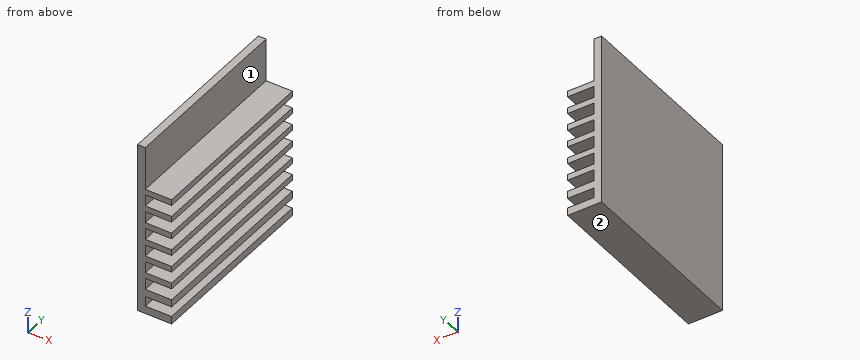
Autodesk Inventor part; units mm, degrees
ref_plane "YZ Plane" through (0, 0, 0) normal (1, 0, 0) x (0, 1, 0)
ref_plane "XZ Plane" through (0, 0, 0) normal (0, 1, 0) x (-1, 0, 0)
ref_plane "XY Plane" through (0, 0, 0) normal (0, 0, 1) x (1, 0, 0)
sketch "Sketch1" plane through (0, 0, 0) normal (0, 1, 0) x (-1, 0, 0)
  line L0 (-10, -20) -> (10, -20)
  line L1 (10, -20) -> (10, 20)
  line L2 (10, 20) -> (-10, 20)
  line L3 (-10, 20) -> (-10, -20)
  line L4 (-10, -20) -> (10, 20) construction
  line L5 (10, -20) -> (-10, 20) construction
  point P0 (0, 0)
  dimension "d0" = 20
  dimension "d1" = 40
extrude "Extrusion1" add sketch "Sketch1" along normal blind 40
sketch "Sketch2" plane through (0, 0, 0) normal (0, -1, 0) x (1, 0, 0)
  line L0 (10, -20) -> (-10, -20)
  line L1 (10, 20) -> (10, -20)
  line L2 (-10, 20) -> (10, 20)
  line L3 (-10, -20) -> (-10, 20)
  line L4 (10, 20) -> (10, -20)
  line L5 (10, 18.3) -> (-5.8, 18.3)
  line L6 (-5.8, 18.3) -> (-5.8, 16.1)
  line L7 (-5.8, 16.1) -> (10, 16.1)
  line L8 (10, 16.1) -> (10, 18.3)
  point P0 (0, 0)
  dimension "d4" = 1.7
  dimension "d5" = 4.2
  dimension "d6" = 2.2
extrude "Extrusion2" cut sketch "Sketch2" against normal through all contours L7 L6 L5 L1
mirror "Mirror1" about plane through (0, 0, 0) normal (0, 0, 1) of "Extrusion2"
sketch "Sketch3" plane through (0, 0, 0) normal (0, -1, 0) x (1, 0, 0)
  line L0 (-5.8, -16.1) -> (10, -16.1)
  line L1 (10, 16.1) -> (10, -16.1)
  line L2 (10, 16.1) -> (-5.8, 16.1)
  line L3 (-5.8, 16.1) -> (-5.8, 18.3)
  line L4 (-5.8, 18.3) -> (10, 18.3)
  line L5 (10, 20) -> (10, 18.3)
  line L6 (-10, 20) -> (10, 20)
  line L7 (-10, -20) -> (-10, 20)
  line L8 (10, -20) -> (-10, -20)
  line L9 (10, -18.3) -> (10, -20)
  line L10 (10, -18.3) -> (-5.8, -18.3)
  line L11 (-5.8, -18.3) -> (-5.8, -16.1)
  line L12 (10, 14.8) -> (-5.8, 14.8)
  line L13 (-5.8, 14.8) -> (-5.8, 12.28)
  line L14 (-5.8, 12.28) -> (10, 12.28)
  line L15 (10, 12.28) -> (10, 14.8)
  point P0 (0, 0)
  dimension "d9" = 1.3
  dimension "d10" = 2.52
extrude "Extrusion3" cut sketch "Sketch3" against normal through all contours L14 L13 L12 L1
pattern_linear "Rectangular Pattern1" count 8 spacing 3.82 along (0, 0, -1) of "Extrusion3"
sketch "Sketch4" plane through (-10, 0, -20) normal (-1, 0, 0) x (0, 0, 1)
  line L0 (0, 0) -> (40, 0)
  line L1 (40, 0) -> (40, 40)
  line L2 (0, 40) -> (40, 40)
  line L3 (0, 0) -> (0, 40)
  point P0 (20, 0)
extrude "Extrusion4" cut sketch "Sketch4" against normal blind 2.5
sketch "Sketch5" plane through (10, 0, 20) normal (1, 0, 0) x (0, 0, -1)
  line L0 (-7.9901, -7.3422) -> (53.3048, -7.3422)
  line L1 (53.3048, -7.3422) -> (53.3048, 101.8937)
  line L2 (53.3048, 101.8937) -> (-7.9901, 101.8937)
  line L3 (-7.9901, 101.8937) -> (-7.9901, -7.3422)
  point P0 (20, 0)
extrude "Extrusion5" cut sketch "Sketch5" against normal blind 10
sketch "Sketch8" plane through (0, 0, 20) normal (1, 0, 0) x (0, 0, -1)
  line L0 (0, 0) -> (40, 0)
  line L1 (0, 40) -> (0, 0)
  line L2 (40, 40) -> (0, 40)
  line L3 (40, 0) -> (40, 40)
  line L4 (0, 0) -> (0, 40)
  line L5 (12.84, 0) -> (11.54, 0)
  line L6 (0, 40) -> (11.54, 40)
  line L7 (11.54, 40) -> (11.54, 0)
  line L8 (11.54, 0) -> (0, 0)
  line L9 (0, 0) -> (0, 40)
  point P0 (20, 0)
extrude "Extrusion8" cut sketch "Sketch8" against normal up to surface (5.8 mm away) contours L1 L2 L7 L0
sketch "Sketch9" plane through (-5.8, 0, 20) normal (0, 0, 1) x (1, 0, 0)
  line L0 (0, 0) -> (0, 40)
  line L1 (-1.7, 40) -> (0, 40)
  line L2 (-1.7, 40) -> (-1.7, 0)
  line L3 (-1.7, 0) -> (0, 0)
  point P0 (5.8, 0)
extrude "Extrusion9" cut sketch "Sketch9" against normal blind 2
properties part number "BMS_Heatsink"
Work out the finished part from the listing and answer in its coordinate system (mm). Face numbers are marked on the shaded views. A direction names the side the tool comes from. Coordinates: 2 decimals unless noted, no trailing zeros. Write each loop counter-clockwise with the first axis right and the second up, starting at its lowest first coordinate (ties: lowest second). Pieces come first, ordered by that corner, then holes.
Q1. Each of these flat-tipped pins is pushed along its axis until it touches: pin 1 Ø0.7 at (y, z) = (28.5, -17) entering from +X; pin 2 Ø1.7 at (x, y) = (-3, 15) entering from +Z. Where does it stop, or does it pass through?
Q2. A cutting plane is placed at A-A, the plane x = -0.75. State how many separate pieces and enclosed holes the cut face has, then the cut area to 3 significant figures.
Q3. Which of the six approach directions +Z, -Z, +X, -X, +Y, -Y give full straight-line access (tool end or side, diameter ignored) to the marked faces 1 and 2?
Q4. A cutting plane is placed at C-C, the plane z = 14.5. Give the vertices of the cut face in (x, y).
Q5. Find the intervals of material crossed by line 1 (X direction, y = 38, z = 15.5), in increasing order.
Findings below:
1. pin 1: stops at x = -5.8
1. pin 2: stops at z = 8.46
2. separate pieces: 8
2. enclosed holes: 0
2. area: 446 mm2
3. face 1: +Z, +X, +Y, -Y
3. face 2: -Z, +X, -X, +Y, -Y
4. outline: (-7.5, 0) - (-5.8, 0) - (-5.8, 40) - (-7.5, 40) - close
5. line 1: x = -7.5 to -5.8
